Build history of the part. All positions in model axes, mm. A direction names the side the tool comes from. Give positions to 0.01 mm unless a question says otherwise; leave off trailing zeros. Write each loop counter-clockwise with the first axis right and the second up, starting at its lowest first coordinate (ties: lowest second). Pieces come first, ordered by that corner, then holes. Notation, with made-up numbers: M 63,18 L 72,18 A36 ccw 72,55 Z; hole C -30.5,80.25 d3. An arc over 180 degrees is marked long. One line per item, written item: value. Start each with the question number.
from build123d import *

# Parameters (mm, degrees)
BOSS_EXTRUDE1_DEPTH     = 55
SKETCH2_W               = 44
SKETCH2_H               = 38
BOSS_EXTRUDE2_DEPTH     = 2
CUT_EXTRUDE1_DEPTH      = 84.360662185
CUT_EXTRUDE1_DEPTH_BACK = 84.360662185
SKETCH3_R               = 4


with BuildPart() as part:
    # Sketch1 → Boss-Extrude1 (new body)
    with BuildSketch(Plane.XY):
        Polygon((0, 0), (0, -42), (-44, -42), (-44, 0), (-42, 0), (-42, -40), (-2, -40), (-2, 0), align=None)
    extrude(amount=BOSS_EXTRUDE1_DEPTH)

    # Sketch2 → Boss-Extrude2 (add)
    with BuildSketch(Plane.XY.offset(55)):
        with Locations((-22, -23)):
            Rectangle(SKETCH2_W, SKETCH2_H)
    extrude(amount=BOSS_EXTRUDE2_DEPTH)

    # Sketch3 → Cut-Extrude1 (cut, two sides: drawn at the far end of the back side and taken through both)
    with BuildSketch(Plane.XY.offset(57).offset(-CUT_EXTRUDE1_DEPTH_BACK)):
        with Locations((-22, -27)):
            Circle(SKETCH3_R)
    extrude(amount=CUT_EXTRUDE1_DEPTH + CUT_EXTRUDE1_DEPTH_BACK, mode=Mode.SUBTRACT)


solid = part.part
1) Band-saw the part on B-B (y = -27). List the corners of the cut face in (x, z), then the cut area to 3 significant figures.
2) Band-saw the part on A-A (x = -22). List the corners of the cut face in (y, z).
3) Drop flat-ended pins along their axis: P1, Ø5, axis at x = -36.5, z = 48, coming from the +Y side; P2, Ø1, axis at x = -42.5, y = -2.5, coming from the +Z side; P3, Ø0.6, axis at x = -25, z = 55.5, coming from the +Y side. Give the stop position or say it passes through.
4) Band-saw the part on D-D (y = -32). List the corners of the cut face in (x, z).
5) Mould opens along X. For faces 4 (the face through (-22, -22, 55)), 5 (the face through (-43, -2, 55)), 6 (the face through (0, -21, 28)), 7 (the face through (-2, -20, 27)) say: released by +X, released by -X, zero draft, split by the parting line, or undercut.
6) Band-saw the part on C-C (z = 33). List the corners of the cut face in (x, y), then the cut area to 3 significant figures.
7) Probe line 1 along X through (y, z) = (-29.5, 34); line 2 along X through (y, z) = (-27, 56.4); line 3 along Y through (x, z) = (-22, 55.65). List the from-to ranges inside material, lowest first. Write a range as from..to.
8) Tool access for faces 1 (the face through (-1, -2, 55)), 2 (the face through (-44, -21, 28)), 3 (the face through (-22, -40, 27)): list every direction of +Z, -Z, +X, -X, +Y, -Y with a clear straight run to the whole face (end or side of a thin tool).
Model answer:
1. outline: M -44,0 L -42,0 L -42,55 L -26,55 L -26,57 L -44,57 Z; M -18,55 L -2,55 L -2,0 L 0,0 L 0,57 L -18,57 Z
1. area: 292 mm²
2. outline: M -42,0 L -40,0 L -40,55 L -31,55 L -31,57 L -42,57 Z; M -23,55 L -4,55 L -4,57 L -23,57 Z
3. P1: stops at y = -40
3. P2: stops at z = 55
3. P3: stops at y = -4
4. outline: M -44,0 L -42,0 L -42,55 L -2,55 L -2,0 L 0,0 L 0,57 L -44,57 Z
5. face 4: undercut
5. face 5: zero draft
5. face 6: released by +X
5. face 7: undercut
6. outline: M -44,-42 L 0,-42 L 0,0 L -2,0 L -2,-40 L -42,-40 L -42,0 L -44,0 Z
6. area: 248 mm²
7. line 1: x = -44..-42, -2..0
7. line 2: x = -44..-26, -18..0
7. line 3: y = -42..-31, -23..-4
8. face 1: +Z, +X, -X, +Y
8. face 2: +Z, -Z, -X, +Y, -Y
8. face 3: -Z, +Y
